The listing builds one solid part. Answer for the finished solid, in the listing's coordinates (mm). Face numbers are marked on the shaded views. A direction names the side the tool comes from. Round coordinates to 2 decimals unless told otherwise and drop trailing zeros. Order: outer loops, then holes, each group sorted by start corner. A loop starts at its lowest first (then second) coordinate and runs counter-clockwise, first axis right, second up. Notation, with made-up numbers: (55.25, 87) - (70.25, 87) arc R13 ccw to (70.25, 102) - close; hole circle Ø4 at (38.25, -25.75). An arc over 180 degrees is marked (long way). Write item = value, one per line.
from build123d import *

# Parameters (mm, degrees)
F1_DEPTH      = 2.75
F2_DEPTH      = 6.75
F2_DEPTH_BACK = 4
F3_DEPTH      = 6.75
F4_DEPTH      = 4.75


with BuildPart() as f1:
    # F0 (on Top) → F1 (new body)
    with BuildSketch(Plane.XY):
        with BuildLine():
            ThreePointArc((2.312466216, 9.8), (1.3919410963, 8.673344038), (1.34e-08, 8.25))
            ThreePointArc((1.34e-08, 8.25), (-1.3919410851, 8.6733440305), (-2.312466216, 9.8))
            Line((-2.312466216, 9.8), (-8.5, 9.8))
            Line((-8.5, 9.8), (-8.5, 11.9319948039))
            ThreePointArc((-8.5, 11.9319948039), (-13.02204861, 6.7118365594), (-14.65, 0))
            ThreePointArc((-14.65, 0), (-14.1933462479, -3.6292454155), (-12.8518536129, -7.0322371059))
            ThreePointArc((-12.8518536129, -7.0322371059), (-10.2873209178, -6.9119317152), (-8.9690606516, -9.1149957636))
            ThreePointArc((-8.9690606516, -9.1149957636), (-9.1731996175, -10.104451226), (-9.7522783412, -10.9323175565))
            ThreePointArc((-9.7522783412, -10.9323175565), (0, -14.65), (9.7522783412, -10.9323175565))
            ThreePointArc((9.7522783412, -10.9323175565), (9.511883066, -7.5595357357), (12.8518536129, -7.0322371059))
            ThreePointArc((12.8518536129, -7.0322371059), (14.1933462479, -3.6292454155), (14.65, 0))
            ThreePointArc((14.65, 0), (13.02204861, 6.7118365594), (8.5, 11.9319948039))
            Line((8.5, 11.9319948039), (8.5, 9.8))
            Line((8.5, 9.8), (2.312466216, 9.8))
        make_face()
        with BuildLine():
            ThreePointArc((1.34e-08, 8.25), (5.8336309495, 5.8336309401), (8.25, 0))
            ThreePointArc((8.25, 0), (-5.8336309495, -5.8336309401), (1.34e-08, 8.25))
        make_face(mode=Mode.SUBTRACT)
        with BuildLine():
            ThreePointArc((9.7522783412, -10.9323175565), (11.4690606516, -9.1149957636), (12.8518536129, -7.0322371059))
            ThreePointArc((12.8518536129, -7.0322371059), (9.511883066, -7.5595357357), (9.7522783412, -10.9323175565))
        make_face()
        with BuildLine():
            ThreePointArc((-8.9690606516, -9.1149957636), (-10.2873209178, -6.9119317152), (-12.8518536129, -7.0322371059))
            ThreePointArc((-12.8518536129, -7.0322371059), (-11.4690606516, -9.1149957636), (-9.7522783412, -10.9323175565))
            ThreePointArc((-9.7522783412, -10.9323175565), (-9.1731996175, -10.104451226), (-8.9690606516, -9.1149957636))
        make_face()
        with BuildLine():
            Line((8.5, 14.225), (8.5, 11.9319948039))
            ThreePointArc((8.5, 11.9319948039), (13.02204861, 6.7118365594), (14.65, 0))
            Line((14.65, 0), (14.65, 9.8))
            Line((14.65, 9.8), (14.65, 14.225))
            ThreePointArc((14.65, 14.225), (13.7493533521, 16.3993533521), (11.575, 17.3))
            ThreePointArc((11.575, 17.3), (9.4006466479, 16.3993533521), (8.5, 14.225))
        make_face()
        with BuildLine():
            ThreePointArc((-14.65, 0), (-13.02204861, 6.7118365594), (-8.5, 11.9319948039))
            Line((-8.5, 11.9319948039), (-8.5, 14.225))
            ThreePointArc((-8.5, 14.225), (-9.4006466479, 16.3993533521), (-11.575, 17.3))
            ThreePointArc((-11.575, 17.3), (-13.7493533521, 16.3993533521), (-14.65, 14.225))
            Line((-14.65, 14.225), (-14.65, 9.8))
            Line((-14.65, 9.8), (-14.65, 0))
        make_face()
        with BuildLine():
            ThreePointArc((-2.312466216, 9.8), (-1.3919410851, 8.6733440305), (1.34e-08, 8.25))
            ThreePointArc((1.34e-08, 8.25), (1.3919410963, 8.673344038), (2.312466216, 9.8))
            Line((2.312466216, 9.8), (0, 9.8))
            Line((0, 9.8), (-2.312466216, 9.8))
        make_face()
        with BuildLine():
            ThreePointArc((2.5, 10.75), (-0.4841665313, 13.2026684998), (-2.312466216, 9.8))
            Line((-2.312466216, 9.8), (0, 9.8))
            Line((0, 9.8), (2.312466216, 9.8))
            ThreePointArc((2.312466216, 9.8), (2.4526684998, 10.2658334687), (2.5, 10.75))
        make_face()
    extrude(amount=F1_DEPTH)

    # F0 (on Top) → F2 (join, two sides)
    with BuildSketch(Plane.XY) as f2_sk:
        with BuildLine():
            ThreePointArc((-12.8518536129, -7.0322371059), (-14.1933462479, -3.6292454155), (-14.65, 0))
            Line((-14.65, 0), (-17.4, 0))
            ThreePointArc((-17.4, 0), (0, -17.4), (17.4, 0))
            Line((17.4, 0), (14.65, 0))
            ThreePointArc((14.65, 0), (14.1933462479, -3.6292454155), (12.8518536129, -7.0322371059))
            ThreePointArc((12.8518536129, -7.0322371059), (13.6721247, -7.9332560298), (13.9690606516, -9.1149957636))
            ThreePointArc((13.9690606516, -9.1149957636), (12.458516114, -11.4108567977), (9.7522783412, -10.9323175565))
            ThreePointArc((9.7522783412, -10.9323175565), (0, -14.65), (-9.7522783412, -10.9323175565))
            ThreePointArc((-9.7522783412, -10.9323175565), (-13.4262382372, -10.6704557915), (-12.8518536129, -7.0322371059))
        make_face()
        with BuildLine():
            ThreePointArc((-9.7522783412, -10.9323175565), (-11.4690606516, -9.1149957636), (-12.8518536129, -7.0322371059))
            ThreePointArc((-12.8518536129, -7.0322371059), (-13.4262382372, -10.6704557915), (-9.7522783412, -10.9323175565))
        make_face()
        with BuildLine():
            ThreePointArc((13.9690606516, -9.1149957636), (13.6721247, -7.9332560298), (12.8518536129, -7.0322371059))
            ThreePointArc((12.8518536129, -7.0322371059), (11.4690606516, -9.1149957636), (9.7522783412, -10.9323175565))
            ThreePointArc((9.7522783412, -10.9323175565), (12.458516114, -11.4108567977), (13.9690606516, -9.1149957636))
        make_face()
    extrude(amount=F2_DEPTH)
    extrude(f2_sk.sketch, amount=-F2_DEPTH_BACK)

    # F0 (on Top) → F3 (join, through all)
    with BuildSketch(Plane.XY):
        with BuildLine():
            ThreePointArc((9.7522783412, -10.9323175565), (11.4690606516, -9.1149957636), (12.8518536129, -7.0322371059))
            ThreePointArc((12.8518536129, -7.0322371059), (9.511883066, -7.5595357357), (9.7522783412, -10.9323175565))
        make_face()
        with BuildLine():
            ThreePointArc((-8.9690606516, -9.1149957636), (-10.2873209178, -6.9119317152), (-12.8518536129, -7.0322371059))
            ThreePointArc((-12.8518536129, -7.0322371059), (-11.4690606516, -9.1149957636), (-9.7522783412, -10.9323175565))
            ThreePointArc((-9.7522783412, -10.9323175565), (-9.1731996175, -10.104451226), (-8.9690606516, -9.1149957636))
        make_face()
        with BuildLine():
            ThreePointArc((-9.7522783412, -10.9323175565), (-11.4690606516, -9.1149957636), (-12.8518536129, -7.0322371059))
            ThreePointArc((-12.8518536129, -7.0322371059), (-13.4262382372, -10.6704557915), (-9.7522783412, -10.9323175565))
        make_face()
    extrude(amount=F3_DEPTH)

    # F0 (on Top) → F4 (join)
    with BuildSketch(Plane.XY):
        with BuildLine():
            ThreePointArc((2.5, 10.75), (-0.4841665313, 13.2026684998), (-2.312466216, 9.8))
            Line((-2.312466216, 9.8), (0, 9.8))
            Line((0, 9.8), (2.312466216, 9.8))
            ThreePointArc((2.312466216, 9.8), (2.4526684998, 10.2658334687), (2.5, 10.75))
        make_face()
        with BuildLine():
            ThreePointArc((-2.312466216, 9.8), (-1.3919410851, 8.6733440305), (1.34e-08, 8.25))
            ThreePointArc((1.34e-08, 8.25), (1.3919410963, 8.673344038), (2.312466216, 9.8))
            Line((2.312466216, 9.8), (0, 9.8))
            Line((0, 9.8), (-2.312466216, 9.8))
        make_face()
    extrude(amount=F4_DEPTH)


solid = f1.part
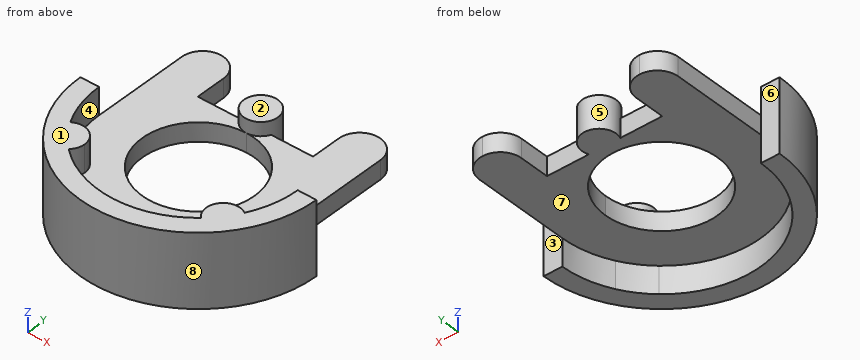
Q1. Section C-C on x = 5 is taken. Determine the outline of the cut face in (y, z), then the cut area to 3 significant figures.
Model answer:
outline = (-16.67, -4) - (-13.77, -4) - (-13.77, 0) - (-6.56, 0) - (-6.56, 2.75) - (-13.77, 2.75) - (-13.77, 6.75) - (-16.67, 6.75) - close; (6.56, 0) - (9.8, 0) - (9.8, 2.75) - (6.56, 2.75) - close
area = 59.9 mm^2
Q2. Section B-B on z = 1.75 is taken. Determine the outline of the cut face in (x, y) (3 decimals), then the cut area to 3 significant figures.
Model answer:
outline = (-17.4, 0) arc R17.4 ccw to (17.4, 0) - (14.65, 0) - (14.65, 14.225) arc R3.075 ccw to (8.5, 14.225) - (8.5, 9.8) - (2.312, 9.8) arc R2.5 ccw (long way) to (-2.312, 9.8) - (-8.5, 9.8) - (-8.5, 14.225) arc R3.075 ccw to (-14.65, 14.225) - (-14.65, 0) - close; hole circle Ø16.5 at (0, 0)
area = 647 mm^2
Q3. Section D-D on z = 5.5 is taken. Determine the outline of the cut face in (x, y) (3 decimals), then the cut area to 3 significant figures.
Model answer:
outline = (-17.4, 0) arc R17.4 ccw to (17.4, 0) - (14.65, 0) arc R14.65 cw to (12.852, -7.032) arc R2.5 ccw to (9.752, -10.932) arc R14.65 cw to (-9.752, -10.932) arc R2.5 ccw to (-12.852, -7.032) arc R14.65 cw to (-14.65, 0) - close
area = 157 mm^2
Q4. Section A-A on y = 10.75 is taken. Determine the outline of the cut face in (x, z).
Model answer:
outline = (-14.65, 0) - (-8.5, 0) - (-8.5, 2.75) - (-14.65, 2.75) - close; (-2.5, 0) - (2.5, 0) - (2.5, 4.75) - (-2.5, 4.75) - close; (8.5, 0) - (14.65, 0) - (14.65, 2.75) - (8.5, 2.75) - close
Q5. Determine the mould class of the marked faces 5, 6, 7 and 8 for opening direction Y: released by +Y, released by -Y, zero draft, split by the parting line, or undercut.
Model answer:
face_5 = undercut
face_6 = released by +Y
face_7 = zero draft
face_8 = released by -Y
Q6. Find the intervals of material crossed by line 1 (X direction, y = -10, z = 3); line 2 (Z direction, x = -9.5, y = -6); line 3 (Y direction, x = -0.5, z = 3), in increasing order. Write a range as from..to.
Model answer:
line_1 = -14.24..-9.13, 9.13..14.24
line_2 = 0..2.75
line_3 = -17.39..-14.64, 8.3..13.2
Q7. For the marked faces 1, 2, 3 and 4, determine the directions among +Z, -Z, +X, -X, +Y, -Y from which every point of the face is accessible in a straight line to the end or side of a thin tool.
Model answer:
face_1 = +Z, +X, -X, +Y, -Y
face_2 = +Z, +X, -X, +Y
face_3 = +Z, -Z, +X, +Y
face_4 = +Z, +Y
Q8. Flat-ended cylindrical pins translate along their axes: P1, Ø4, axis at y = 3.5, z = 4, coming from the -X side; P2, Ø3, axis at y = -5.5, z = 4.5, coming from the -X side; P3, Ø10, axis at x = -9.5, y = 11, coming from the +Z side; P4, Ø3, axis at y = 2.5, z = 5.5, coming from the -X side. Find the tip coordinate at first contact, or state that the pin passes through.
Model answer:
P1 = -14.65
P2 = -16.93
P3 = 2.75
P4 = through
